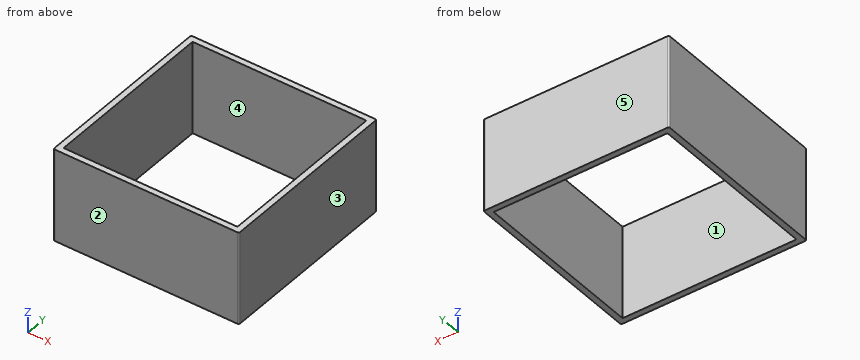
from build123d import *

# Parameters (mm, degrees)
F0_W     = 25.4
F0_H     = 25.4
F1_DEPTH = 12.7
F2_R     = 0.2
F3_T     = -0.8


with BuildPart() as f1:
    # F0 (on Top) → F1 (new body)
    with BuildSketch(Plane.XY):
        Rectangle(F0_W, F0_H)
    extrude(amount=F1_DEPTH)

    # F2
    f2_edges = [f1.edges().sort_by_distance(p)[0] for p in [
        (12.7, -12.7, 6.35),
        (12.7, 12.7, 6.35),
        (-12.7, -12.7, 6.35),
        (-12.7, 12.7, 6.35),
    ]]
    fillet(f2_edges, radius=F2_R)

    # F3
    f3_openings = [f1.faces().sort_by_distance(p)[0] for p in [
        (0, 0, 12.7),
        (0, 0, 0),
    ]]
    offset(amount=F3_T, openings=f3_openings)


solid = f1.part
Part model, mm, in its own coordinate system. Face numbers are marked on the shaded views. A direction names the side the tool comes from. Coordinates: 2 decimals unless noted, no trailing zeros. Loops run counter-clockwise (first coordinate to the right, second up) from the corner with the lowest first, then second, coordinate; pieces in that order, holes last. Notation, with made-up numbers: M 76,76 L 129,76 A6 ccw 129,86 Z; hole C -9,-37 d11. An arc over 180 degrees is marked long. Use a Markdown table: item, result. Add a question column.
Q1. Which spindle directions (+Z, -Z, +X, -X, +Y, -Y) get a long thin tool onto all of the face, cutting with end or side? Do the marked faces 1 and 2. Say none if no direction does.
Q2. Cut at C-C (z = 8.75). Write the cut outline in (x, y), and give its area (3 significant figures).
Q3. Probe L1, parallel to Y at x = 9, z = 10.25. List the from-to ranges inside material, lowest first.
Q4. Mould opens along X. For the marked faces 3, 4 and 5 say: +X half, -X half, draft (parallel to the pull), parting line (faces both ways), or undercut.
Q5. Cut at A-A (x = -3.25). Write the cut outline in (y, z).
Q6. Pin check, flat tip, straight feed: P1, Ø5, axis at x = 2, y = 8.5, coming from the -Z side. Stop position of the tip, or through.
Worked out:
| question | item | result |
|---|---|---|
| 1 | face 1 | +Z, -Z |
| 1 | face 2 | +Z, -Z, +X, -X, -Y |
| 2 | outline | M -12.7,-12.5 A0.2 ccw -12.5,-12.7 L 12.5,-12.7 A0.2 ccw 12.7,-12.5 L 12.7,12.5 A0.2 ccw 12.5,12.7 L -12.5,12.7 A0.2 ccw -12.7,12.5 Z; hole M -11.9,-11.9 L 11.9,-11.9 L 11.9,11.9 L -11.9,11.9 Z |
| 2 | area | 78.7 mm2 |
| 3 | L1 | y = -12.7 to -11.9, 11.9 to 12.7 |
| 4 | face 3 | +X half |
| 4 | face 4 | undercut |
| 4 | face 5 | draft |
| 5 | outline | M -12.7,0 L -11.9,0 L -11.9,12.7 L -12.7,12.7 Z; M 11.9,0 L 12.7,0 L 12.7,12.7 L 11.9,12.7 Z |
| 6 | P1 | passes through |
